Here's how the part is built. I have some questions about the finished solid (model axes, mm). A direction names the side the tool comes from. Round coordinates to 2 decimals unless told otherwise and drop trailing zeros. Write each loop counter-clockwise with the first axis right and the second up, starting at its lowest first coordinate (ties: lowest second). Pieces come first, ordered by that corner, then holes. Notation, with made-up numbers: (86.5, 44) - (127.5, 44) arc R9 ccw to (127.5, 57) - close; hole circle Ø8 at (55, 73). An arc over 180 degrees is marked (long way). Return JSON: item names as keys, results as strings. Group by question number.
```python
from build123d import *

# Parameters (mm, degrees)
F0_W     = 2.5
F0_H     = 4.5
F0_W_2   = 1
F1_DEPTH = 20
F0_H_2   = 1
F2_DEPTH = 22
F3_R     = 0.5
F4_W     = 4
F4_H     = 10
F5_DEPTH = 12.5


with BuildPart() as f1:
    # F0 (on Front) → F1 (new body)
    with BuildSketch(Plane.XZ):
        Rectangle(F0_W, F0_H)
        with Locations((1.75, 0)):
            Rectangle(F0_W_2, F0_H)
        with Locations((-1.75, 0)):
            Rectangle(F0_W_2, F0_H)
    extrude(amount=F1_DEPTH)

    # F0 (on Front) → F2 (join)
    with BuildSketch(Plane.XZ):
        with Locations((0, 2.75)):
            Rectangle(F0_W, F0_H_2)
        Rectangle(F0_W, F0_H)
        with Locations((0, -2.75)):
            Rectangle(F0_W, F0_H_2)
    extrude(amount=-F2_DEPTH)

    # F3
    f3_edges = [f1.edges().sort_by_distance(p)[0] for p in [
        (-2.25, -10, 2.25),
        (-1.25, 11, 3.25),
        (1.25, 11, 3.25),
        (-1.25, 11, -3.25),
        (-2.25, -10, -2.25),
        (1.25, 11, -3.25),
        (2.25, -10, -2.25),
        (2.25, -10, 2.25),
    ]]
    fillet(f3_edges, radius=F3_R)

    # F4 (on Right) → F5 (cut, symmetric)
    with BuildSketch(Plane.YZ):
        Rectangle(F4_W, F4_H)
    extrude(amount=F5_DEPTH, both=True, mode=Mode.SUBTRACT)

    # F5_face (on face) → F6 section 0
    with BuildSketch(Plane.XZ.offset(-2)):
        with BuildLine():
            Line((1.25, -2.75), (1.25, 2.75))
            ThreePointArc((1.25, 2.75), (1.1035533906, 3.1035533906), (0.75, 3.25))
            Line((0.75, 3.25), (-0.75, 3.25))
            ThreePointArc((-0.75, 3.25), (-1.1035533906, 3.1035533906), (-1.25, 2.75))
            Line((-1.25, 2.75), (-1.25, -2.75))
            ThreePointArc((-1.25, -2.75), (-1.1035533906, -3.1035533906), (-0.75, -3.25))
            Line((-0.75, -3.25), (0.75, -3.25))
            ThreePointArc((0.75, -3.25), (1.1035533906, -3.1035533906), (1.25, -2.75))
        make_face()
    # F5_face1 (on face) → F6 section 1
    with BuildSketch(Plane(origin=(0, -2, 0), x_dir=(-1, 0, 0), z_dir=(0, 1, 0))):
        with BuildLine():
            ThreePointArc((-2.25, -1.75), (-2.1035533906, -2.1035533906), (-1.75, -2.25))
            Line((-1.75, -2.25), (1.75, -2.25))
            ThreePointArc((1.75, -2.25), (2.1035533906, -2.1035533906), (2.25, -1.75))
            Line((2.25, -1.75), (2.25, 1.75))
            ThreePointArc((2.25, 1.75), (2.1035533906, 2.1035533906), (1.75, 2.25))
            Line((1.75, 2.25), (-1.75, 2.25))
            ThreePointArc((-1.75, 2.25), (-2.1035533906, 2.1035533906), (-2.25, 1.75))
            Line((-2.25, 1.75), (-2.25, -1.75))
        make_face()
    loft()


solid = f1.part
```
1) Will these pins go through, and if not, where does the flat tip stop? pin 1 Ø1.8 at (x, y) = (-0.5, -15) entering from +Z; pin 2 Ø1 at (x, y) = (-0.5, -9) entering from -Z; pin 3 Ø3 at (y, z) = (11.5, 2.5) entering from -X.
2) Imagine slicing it at A-A (y = 15). Please give me the cut outline in (x, z).
3) I need wall thicknesses on line 1 along Z through (x, y) = (-0.45, -5); line 2 along X through (y, z) = (14, -1.25). Which ranges of each line are inside material? Lowest first, please.
4) Imagine slicing it at B-B (y = -15.5). Please give me the cut outline in (x, z).
5) For faces 1 (the flat face through (1.25, 12, 0)), 2 (the flat face through (0, -11, -2.25)), 3 (the flat face through (-1.25, 12, 0)), which set-ups out of +Z, -Z, +X, -X, +Y, -Y let a thin tool reach every point of the face, with its end or its side?
Results found:
{
 "1": {"pin 1": "stops at z = 2.25", "pin 2": "stops at z = -2.25", "pin 3": "stops at x = -1.25"},
 "2": {"outline": "(-1.25, -2.75) arc R0.5 ccw to (-0.75, -3.25) - (0.75, -3.25) arc R0.5 ccw to (1.25, -2.75) - (1.25, 2.75) arc R0.5 ccw to (0.75, 3.25) - (-0.75, 3.25) arc R0.5 ccw to (-1.25, 2.75) - close"},
 "3": {"line 1": "z = -2.25 to 2.25", "line 2": "x = -1.25 to 1.25"},
 "4": {"outline": "(-2.25, -1.75) arc R0.5 ccw to (-1.75, -2.25) - (1.75, -2.25) arc R0.5 ccw to (2.25, -1.75) - (2.25, 1.75) arc R0.5 ccw to (1.75, 2.25) - (-1.75, 2.25) arc R0.5 ccw to (-2.25, 1.75) - close"},
 "5": {"face 1": "+Z, -Z, +X, +Y", "face 2": "-Z, +X, -X, -Y", "face 3": "+Z, -Z, -X, +Y"}
}
